Check sheet for the modelled part. Datum: model origin and axes. Units: mm. A direction names the side the tool comes from. Round coordinates to 2 decimals unless told otherwise and drop trailing zeros. Order: outer loops, then holes, each group sorted by start corner. A loop starts at its lowest first (then second) coordinate and runs counter-clockwise, first axis right, second up. Notation, with made-up numbers: (-13.75, 30) -> (18.25, 30) arc R23 ccw to (18.25, 40) -> close; hole circle Ø2 at (38.25, 44.25). An arc over 180 degrees is marked (long way). Answer in a Markdown table with one row per item.
```python
from build123d import *

# Parameters (mm, degrees)
BOSS_EXTRUDE1_DEPTH = 9
CUT_EXTRUDE1_DEPTH  = 265.443626141
SKETCH5_R           = 1.6
SKETCH5_W           = 9
SKETCH5_H           = 20
CUT_EXTRUDE2_DEPTH  = 265.443626141


with BuildPart() as part:
    # Sketch2 → Boss-Extrude1 (new body)
    with BuildSketch(Plane(origin=(0, -59.966770125, 10.573759519), x_dir=(1, 0, 0), z_dir=(0, 0.9848077530122079, -0.1736481776669316))):
        Polygon((-80, -33.247729948), (-89, -33.247729948), (-89, -48.247729948), (-80, -48.247729948), (-80, -75.240683317), (242, -75.240683317), (242, -48.247729948), (251, -48.247729948), (251, -33.247729948), (242, -33.247729948), (242, -4.497729948), (251, -4.497729948), (251, 10.502270052), (242, 10.502270052), (242, 39.252270052), (251, 39.252270052), (251, 54.252270052), (242, 54.252270052), (242, 81.245223421), (-80, 81.245223421), (-80, 54.252270052), (-89, 54.252270052), (-89, 39.252270052), (-80, 39.252270052), (-80, 10.502270052), (-89, 10.502270052), (-89, -4.497729948), (-80, -4.497729948), align=None)
    extrude(amount=BOSS_EXTRUDE1_DEPTH)

    # Sketch4 → Cut-Extrude1 (cut, through all)
    with BuildSketch(Plane(origin=(0, -51.103500347, 9.01092592), x_dir=(1, 0, 0), z_dir=(0, 0.9848077530122079, -0.17364817766693172))):
        Polygon((-80, -17.172729948), (-76.2, -17.172729948), (-76.2, -16.122729948), (-74, -16.122729948), (-74, -17.172729948), (-71, -17.172729948), (-71, -20.572729948), (-74, -20.572729948), (-74, -21.622729948), (-76.2, -21.622729948), (-76.2, -20.572729948), (-80, -20.572729948), align=None)
        Polygon((-80, 23.177270052), (-80, 26.577270052), (-76.2, 26.577270052), (-76.2, 27.627270052), (-74, 27.627270052), (-74, 26.577270052), (-71, 26.577270052), (-71, 23.177270052), (-74, 23.177270052), (-74, 22.127270052), (-76.2, 22.127270052), (-76.2, 23.177270052), align=None)
        Polygon((242, 23.177270052), (238.2, 23.177270052), (238.2, 22.127270052), (236, 22.127270052), (236, 23.177270052), (233, 23.177270052), (233, 26.577270052), (236, 26.577270052), (236, 27.627270052), (238.2, 27.627270052), (238.2, 26.577270052), (242, 26.577270052), align=None)
        Polygon((242, -17.172729948), (242, -20.572729948), (238.2, -20.572729948), (238.2, -21.622729948), (236, -21.622729948), (236, -20.572729948), (233, -20.572729948), (233, -17.172729948), (236, -17.172729948), (236, -16.122729948), (238.2, -16.122729948), (238.2, -17.172729948), align=None)
    extrude(amount=-CUT_EXTRUDE1_DEPTH, mode=Mode.SUBTRACT)

    # Sketch5 → Cut-Extrude2 (cut, through all)
    with BuildSketch(Plane(origin=(0, -51.103500347, 9.01092592), x_dir=(1, 0, 0), z_dir=(0, 0.9848077530122078, -0.1736481776669317))):
        with Locations(Location((91.5, -21.542669597, 0), (0, 0, 270))):
            Circle(SKETCH5_R)
        with Locations(Location((91.5, 21.542669597, 0), (0, 0, 270))):
            Circle(SKETCH5_R)
        with Locations((91.5, -43.085339194)):
            Rectangle(SKETCH5_W, SKETCH5_H)
        with Locations((91.5, 0)):
            Rectangle(SKETCH5_W, SKETCH5_H)
        with Locations((91.5, 43.085339194)):
            Rectangle(SKETCH5_W, SKETCH5_H)
    cut_extrude2 = extrude(amount=-CUT_EXTRUDE2_DEPTH, mode=Mode.SUBTRACT)

    # Mirror1: Cut-Extrude2 across plane
    add(cut_extrude2.mirror(Plane.ZY.offset(-81)), mode=Mode.SUBTRACT)


solid = part.part
```
(1) Section check B-B on x = 198.5. Record the boundary of the cut face in (y, z), plus the area to 3 significant figures.
Solutions:
| item | result |
|---|---|
| outline | (-74.07, -69.44) -> (-65.21, -71) -> (-38.04, 83.11) -> (-46.9, 84.67) -> close |
| area | 1,410 mm^2 |
(2) Draft check along X on faces 1 (the flat face through (-80, -61, -23)), 2 (the flat face through (87, -55, 10)), 3 (the flat face through (-84.563, -62.413, -28.853)). Enter one of: pulls with the +X half, pulls with the -X half, needs draft (parallel to the pull), parting line crosses it, or undercut.
Solutions:
| item | result |
|---|---|
| face 1 | pulls with the -X half |
| face 2 | undercut |
| face 3 | needs draft |
(3) Tool access check on faces 4 (the flat face through (246.56, -57.42, -0.54)), 5 (the flat face through (91.44, -61.22, -22.8)), 6 (the flat face through (246.44, -47.22, 57.32)). Record the directions out of +Z, -Z, +X, -X, +Y, -Y that give a thin tool (end or side, any length) a straight path to the whole face; none if there is none.
Solutions:
| item | result |
|---|---|
| face 4 | +X, -Y |
| face 5 | -Y |
| face 6 | +Z, +X, +Y |
(4) Section check C-C on z = -60.5. Record the boundary of the cut face in (x, y).
Solutions:
| item | result |
|---|---|
| outline | (-80, -72.5) -> (242, -72.5) -> (242, -63.36) -> (-80, -63.36) -> close |
(5) Scan lines: probe 1 along X at (y, z) = (-52.5, 7.5); probe 2 along X at (y, z) = (-66, -44); probe 3 along Y at (x, z) = (221, 21). Record each from-to range of solid material in increasing order. Write a range as from..to.
Solutions:
| item | result |
|---|---|
| probe 1 | -89..66, 75..87, 96..251 |
| probe 2 | -80..242 |
| probe 3 | -58.13..-48.99 |
(6) Depth check by flat-ended pin: pin 1 Ø5 at (x, z) = (89, 39) entering from -Y; pin 2 Ø5 at (x, z) = (-31.5, 31) entering from -Y; pin 3 Ø3.5 at (y, z) = (-55, 23.5) entering from -X; pin 4 Ø5 at (y, z) = (-52.5, -26.5) entering from +X. Enter the tip coordinate at first touch or a pass-through.
Solutions:
| item | result |
|---|---|
| pin 1 | y = -55.4 |
| pin 2 | y = -56.81 |
| pin 3 | x = -80 |
| pin 4 | through |
(7) Section check A-A on z = 5. Record the boundary of the cut face in (x, y).
Solutions:
| item | result |
|---|---|
| outline | (-89, -60.95) -> (66, -60.95) -> (66, -51.81) -> (-89, -51.81) -> close; (75, -60.95) -> (87, -60.95) -> (87, -51.81) -> (75, -51.81) -> close; (96, -60.95) -> (251, -60.95) -> (251, -51.81) -> (96, -51.81) -> close |
